For this review, take the finished solid that the model builds, in its own axes (mm). A direction names the side the tool comes from. Give positions to 0.01 mm unless a question says otherwise; leave off trailing zeros. Write each loop counter-clockwise with the first axis right and the second up, starting at its lowest first coordinate (ties: lowest second). Pieces come first, ordered by that corner, then holes.
1) We need section B-B on x = -31. Give the boundary of the cut face in (y, z) (3 decimals).
2) We need section D-D on y = 0.75. Give the number of separate pieces and of enclosed holes in the cut face, and give its area (3 significant figures).
3) We need section C-C on z = 13. Give the boundary of the cut face in (x, y).
4) For P1, Ø2, axis at x = -33, z = 3.5, coming from the -Y side; P2, Ø3, axis at y = -8.5, z = 12, coming from the +X side; P3, Ø3, axis at y = -3, z = 4, coming from the +X side, all flat-tipped, find the tip position at first contact; note any pin that passes through.
5) Machinability: for faces 1 (the face through (11, 1, -0.975)), 2 (the face through (-33, -5, -7.475)), 3 (the face through (-0.5, -5, 13)), 4 (the face through (8.54, 2.01, 9.77)), which of the approach directions +Z, -Z, +X, -X, +Y, -Y give a long, thin tool a straight path to every point of the face, cutting with its end or side? Answer none if there is none.
6) Draft analysis for pull direction X (two halves, no side actions). For faces 5 (the face through (34.05, -4, 3)), 6 (the face through (-30, 1, -0.975)), 7 (the face through (35, -5, -7.525)), state which applies: pulls with the +X half, pulls with the -X half, needs draft (parallel to the pull), parting line crosses it, or undercut.
7) We need section A-A on y = -5.25. Give the boundary of the cut face in (x, z) (3 decimals).
8) Wall thickness on line 1 along X through (y, z) = (-9.25, -4); line 2 along X through (y, z) = (-4.25, 1); line 3 along X through (y, z) = (-8.25, 1): over which ranges is each line inside the solid? List them lowest first.
from build123d import *

# Parameters (mm, degrees)
SKETCH1_W           = 72.1
SKETCH1_H           = 31.95
BOSS_EXTRUDE1_DEPTH = 2.5
FILLET1_R           = 2
SKETCH2_W           = 2
SKETCH2_H           = 8.4
SKETCH2_W_2         = 9
SKETCH2_H_2         = 2
BOSS_EXTRUDE2_DEPTH = 10.6
BOSS_EXTRUDE4_DEPTH = 9.75
CUT_EXTRUDE1_DEPTH  = 2.5
CUT_EXTRUDE2_DEPTH  = 1
CUT_EXTRUDE4_DEPTH  = 1
SKETCH8_W           = 15
SKETCH8_H           = 7.5
BOSS_EXTRUDE5_DEPTH = 2


with BuildPart() as part:
    # Sketch1 → Boss-Extrude1 (new body)
    with BuildSketch(Plane(origin=(0, 0, 0), x_dir=(1, 0, 0), z_dir=(0, 1, 0))):
        Rectangle(SKETCH1_W, SKETCH1_H)
    extrude(amount=BOSS_EXTRUDE1_DEPTH)

    # Fillet1
    fillet1_edges = [part.edges().sort_by_distance(p)[0] for p in [
        (36.05, 1.25, 15.975),
        (-36.05, 1.25, 15.975),
        (-36.05, 1.25, -15.975),
        (36.05, 1.25, -15.975),
    ]]
    fillet(fillet1_edges, radius=FILLET1_R)

    # Sketch2 → Boss-Extrude2 (add)
    with BuildSketch(Plane.XZ):
        with Locations((35.05, -3.325)):
            Rectangle(SKETCH2_W, SKETCH2_H)
        with Locations((4, -13.725)):
            Rectangle(SKETCH2_W_2, SKETCH2_H_2)
        with Locations((4, 12.975)):
            Rectangle(SKETCH2_W_2, SKETCH2_H_2)
    extrude(amount=BOSS_EXTRUDE2_DEPTH)

    # Sketch2<3> → Boss-Extrude4 (add)
    with BuildSketch(Plane.XZ):
        Polygon((-32.05, 7.475), (-32.05, -0.925), (-32.05, -7.475), (-34.05, -7.475), (-34.05, -0.925), (-34.05, 7.475), align=None)
    extrude(amount=BOSS_EXTRUDE4_DEPTH)

    # Sketch4 → Cut-Extrude1 (cut)
    with BuildSketch(Plane(origin=(0, 2.5, 0), x_dir=(1, 0, 0), z_dir=(0, 1, 0))):
        Polygon((-32.05, 0.975), (-27.375612096, 0.975), (-23.371939519, 11.975), (-28.046327423, 11.975), align=None)
        Polygon((-22.701224192, 0.975), (-18.697551615, 11.975), (-14.023163712, 11.975), (-18.026836288, 0.975), align=None)
        Polygon((-13.352448385, 0.975), (-9.348775808, 11.975), (-4.674387904, 11.975), (-8.678060481, 0.975), align=None)
        Polygon((0, 11.975), (-4.003672577, 0.975), (4.003672577, 0.975), align=None)
        Polygon((8.678060481, 0.975), (4.674387904, 11.975), (9.348775808, 11.975), (13.352448385, 0.975), align=None)
        Polygon((18.026836288, 0.975), (14.023163712, 11.975), (18.697551615, 11.975), (22.701224192, 0.975), align=None)
        Polygon((23.371939519, 11.975), (27.375612096, 0.975), (32.05, 0.975), (28.046327423, 11.975), align=None)
    extrude(amount=-CUT_EXTRUDE1_DEPTH, mode=Mode.SUBTRACT)

    # Sketch3 → Cut-Extrude2 (cut)
    # profile 1 of 6: a face of its own
    with BuildSketch(Plane(origin=(0, 2.5, 0), x_dir=(1, 0, 0), z_dir=(0, 1, 0))):
        Polygon((-29.003846154, -2.45), (-27.294230769, -2.45), (-27.294230769, -10.265384615), (-24.607692308, -10.265384615), (-24.607692308, -11.975), (-29.003846154, -11.975), align=None)
    # profile 2 of 6: a face of its own
    with BuildSketch(Plane(origin=(0, 2.5, 0), x_dir=(1, 0, 0), z_dir=(0, 1, 0))):
        Polygon((-14.585399639, -2.45), (-12.999807692, -2.45), (-9.153173077, -11.975), (-10.979179687, -11.975), (-11.719504207, -10.021153846), (-15.869519231, -10.021153846), (-16.60984375, -11.975), (-18.433942308, -11.975), align=None)
        Polygon((-13.793557692, -5.004882812), (-15.22078125, -8.311538462), (-12.366334135, -8.311538462), align=None, mode=Mode.SUBTRACT)
    # profile 3 of 6: a face of its own
    with BuildSketch(Plane(origin=(0, 2.5, 0), x_dir=(1, 0, 0), z_dir=(0, 1, 0))):
        Polygon((-6.136923077, -2.45), (-4.597124399, -2.45), (-0.275384615, -8.717953726), (-0.275384615, -2.45), (1.434230769, -2.45), (1.434230769, -11.975), (-0.117016226, -11.975), (-4.427307692, -5.726126803), (-4.427307692, -11.975), (-6.136923077, -11.975), align=None)
    # profile 4 of 6: a face of its own
    with BuildSketch(Plane(origin=(0, 2.5, 0), x_dir=(1, 0, 0), z_dir=(0, 1, 0))):
        Polygon((5.244230769, -2.45), (6.953846154, -2.45), (6.953846154, -5.802448918), (9.655649038, -2.45), (11.813656851, -2.45), (8.419230769, -6.662980769), (12.14375, -11.975), (10.084960938, -11.975), (6.953846154, -7.508248197), (6.953846154, -11.975), (5.244230769, -11.975), align=None)
    # profile 5 of 6: a face of its own
    with BuildSketch(Plane(origin=(0, 2.5, 0), x_dir=(1, 0, 0), z_dir=(0, 1, 0))):
        Polygon((15.037884615, -2.45), (16.7475, -2.45), (16.7475, -10.265384615), (19.434038462, -10.265384615), (19.434038462, -11.975), (15.037884615, -11.975), align=None)
    # profile 6 of 6: a face of its own
    with BuildSketch(Plane(origin=(0, 2.5, 0), x_dir=(1, 0, 0), z_dir=(0, 1, 0))):
        Polygon((22.511346154, -2.45), (27.640192308, -2.45), (27.640192308, -4.159615385), (24.220961538, -4.159615385), (24.220961538, -5.991346154), (27.640192308, -5.991346154), (27.640192308, -7.700961538), (24.220961538, -7.700961538), (24.220961538, -10.265384615), (27.640192308, -10.265384615), (27.640192308, -11.975), (22.511346154, -11.975), align=None)
    extrude(amount=-CUT_EXTRUDE2_DEPTH, mode=Mode.SUBTRACT)

    # Sketch7 → Cut-Extrude4 (cut)
    with BuildSketch(Plane(origin=(0, 2.5, 0), x_dir=(1, 0, 0), z_dir=(0, 1, 0))):
        Polygon((-12.366334135, -8.311538462), (-13.793557692, -5.004882812), (-15.22078125, -8.311538462), align=None)
    extrude(amount=-CUT_EXTRUDE4_DEPTH, mode=Mode.SUBTRACT)

    # Sketch8 → Boss-Extrude5 (add)
    with BuildSketch(Plane.ZY.offset(-34.05)):
        with Locations((-3.325, -3.75)):
            Rectangle(SKETCH8_W, SKETCH8_H)
    extrude(amount=BOSS_EXTRUDE5_DEPTH)


solid = part.part
Results list:
1. outline: (0, -15.975) - (2.5, -15.975) - (2.5, -3.86) - (0, -3.86) - close; (0, -0.975) - (2.5, -0.975) - (2.5, 15.975) - (0, 15.975) - close
2. separate pieces: 1
2. enclosed holes: 7
2. area: 1,950 mm2
3. outline: (-36.05, 0) - (-0.5, 0) - (-0.5, -10.6) - (8.5, -10.6) - (8.5, 0) - (36.05, 0) - (36.05, 2.5) - (-36.05, 2.5) - close
4. P1: stops at y = -9.75
4. P2: stops at x = 8.5
4. P3: stops at x = 34.05
5. face 1: +Y, -Y
5. face 2: -Z, -X, -Y
5. face 3: +Z, -Z, -X, -Y
5. face 4: +Y
6. face 5: pulls with the +X half
6. face 6: undercut
6. face 7: needs draft
7. outline: (-34.05, -7.475) - (-32.05, -7.475) - (-32.05, 7.475) - (-34.05, 7.475) - close; (-0.5, -14.725) - (8.5, -14.725) - (8.5, -12.725) - (-0.5, -12.725) - close; (-0.5, 11.975) - (8.5, 11.975) - (8.5, 13.975) - (-0.5, 13.975) - close; (32.05, -10.825) - (34.05, -10.825) - (34.05, -7.525) - (36.05, -7.525) - (36.05, 0.875) - (34.05, 0.875) - (34.05, 4.175) - (32.05, 4.175) - close
8. line 1: x = -34.05 to -32.05, 34.05 to 36.05
8. line 2: x = -34.05 to -32.05, 32.05 to 34.05
8. line 3: x = -34.05 to -32.05
